Geometry: see drawing. Coordinates: mm, zero at the bounding-box minimum. A direction names the side the tool comes from. Coordinates: 2 decimals unless noted, no trailing zeros. Loops run counter-clockwise (first coordinate to the right, second up) from the corner with the lowest first, then second, coordinate; pieces in that order, holes last. Notation, with made-up numbers: (-5.75, -6.5) -> (19.25, -6.5) arc R22 cw to (19.25, 16.5) -> close; hole circle Ø8 at (69.5, -32). An arc over 180 degrees is marked (long way). One line per item, written item: value. Start each with the question number.
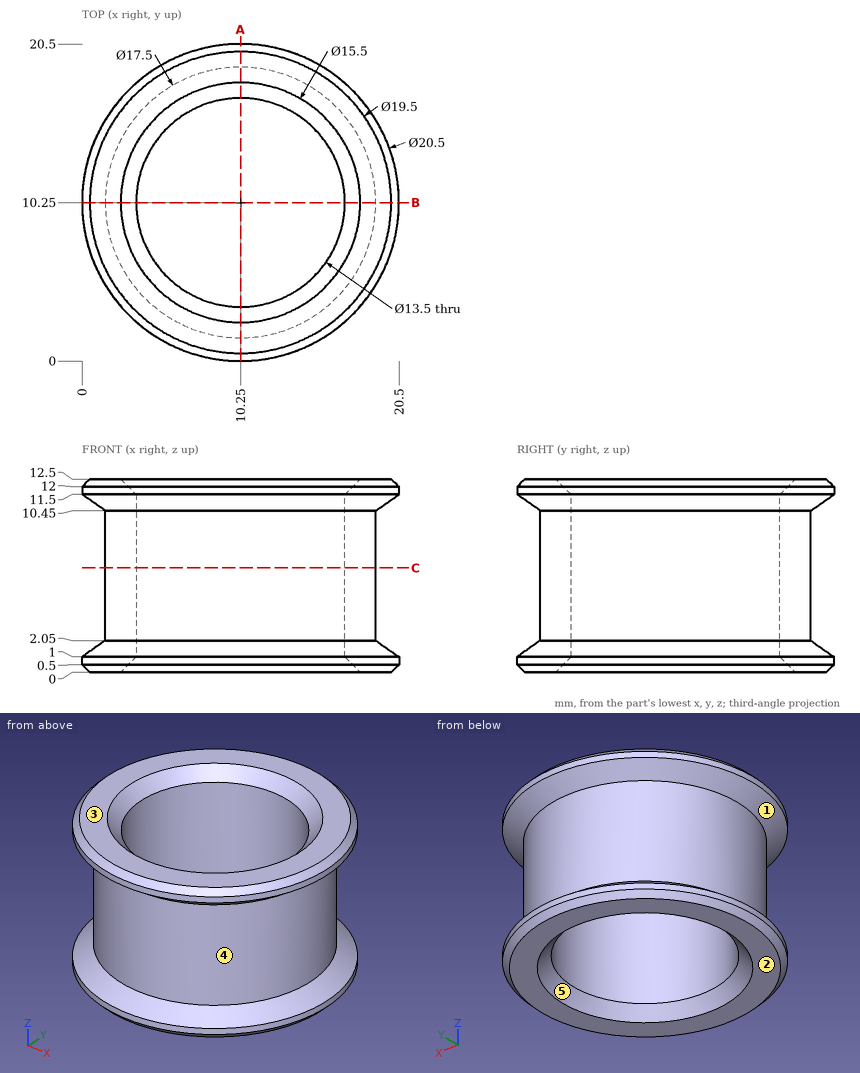
1. Pin query (flat end, axial travel): pin 1 Ø3 at (y, z) = (8, 9) entering from -X; pin 2 Ø6 at (x, z) = (4, 3) entering from +Y; pin 3 Ø1.5 at (x, z) = (18.5, 3.5) entering from +Y; pin 4 Ø5 at (x, y) = (9.5, 17) entering from +Z. Return the tip coordinate at first contact, or that it passes through.
2. Line query: L1, parallel to X at y = 10.25, z = 4.75; L2, parallel to Y at x = 6.25, z = 4.5. Output: solid intervals per line, ascending. Write a range as [from, to].
3. Section A-A on x = 10.25. Return the cut outline in (y, z).
4. Section C-C on z = 6.75. Return the cut outline in (x, y).
5. Set-up query: the marked faces 1 and 2. Return all of +Z, -Z, +X, -X, +Y, -Y with unobstructed straight access to the full face (end or side cutting, diameter ignored); none if empty.
6. Draft query along Z for the marked faces 3, 4 and 5. Return one class per face: released by +Z, released by -Z, zero draft, split by the parting line, or undercut.
Checks:
1. pin 1: x = 1.53
1. pin 2: y = 19.68
1. pin 3: y = 14.76
1. pin 4: z = 12.5
2. L1: [1.5, 3.5], [17, 19]
2. L2: [2.47, 4.81], [15.69, 18.03]
3. outline: (0, 0.5) -> (0.5, 0) -> (2.5, 0) -> (3.5, 1) -> (3.5, 11.5) -> (2.5, 12.5) -> (0.5, 12.5) -> (0, 12) -> (0, 11.5) -> (1.5, 10.45) -> (1.5, 2.05) -> (0, 1) -> close; (17, 1) -> (18, 0) -> (20, 0) -> (20.5, 0.5) -> (20.5, 1) -> (19, 2.05) -> (19, 10.45) -> (20.5, 11.5) -> (20.5, 12) -> (20, 12.5) -> (18, 12.5) -> (17, 11.5) -> close
4. outline: circle Ø17.5 at (10.25, 10.25); hole circle Ø13.5 at (10.25, 10.25)
5. face 1: none
5. face 2: -Z, +X, -X, +Y, -Y
6. face 3: released by +Z
6. face 4: undercut
6. face 5: released by -Z
